from build123d import *

# Parameters (mm, degrees)
F0_W      = 150
F0_H      = 150
F1_DEPTH  = 25
F2_T      = -3
F3_R      = 6.25
F4_DEPTH  = 30
F5_R      = 6.25
F6_DEPTH  = 25
F7_R      = 6.25
F8_DEPTH  = 30
F9_R      = 6.25
F10_DEPTH = 30


with BuildPart() as f1:
    # F0 (on Front) → F1 (new body)
    with BuildSketch(Plane.XZ):
        with Locations((-12.459678, 3.580103)):
            Rectangle(F0_W, F0_H)
    extrude(amount=F1_DEPTH)

    # F2
    f2_openings = [f1.faces().sort_by_distance(p)[0] for p in [
        (-12.459678, 0, 3.580103),
    ]]
    offset(amount=F2_T, openings=f2_openings)

    # F3 (on face) → F4 (join)
    with BuildSketch(Plane.XY.offset(78.580103)):
        with Locations((-74.959678, -12.5)):
            Circle(F3_R)
        with Locations((50.040322, -12.5)):
            Circle(F3_R)
    extrude(amount=F4_DEPTH)

    # F5 (on face) → F6 (cut)
    with BuildSketch(Plane(origin=(0, 0, -71.419897), x_dir=(1, 0, 0), z_dir=(0, 0, -1))):
        with Locations((-74.959678, 12.5)):
            Circle(F5_R)
        with Locations((50.040322, 12.5)):
            Circle(F5_R)
    extrude(amount=-F6_DEPTH, mode=Mode.SUBTRACT)

    # F7 (on face) → F8 (join)
    with BuildSketch(Plane(origin=(-87.459678, 0, 0), x_dir=(0, -1, 0), z_dir=(-1, 0, 0))):
        with Locations((12.5, 66.080103)):
            Circle(F7_R)
        with Locations((12.5, -58.919897)):
            Circle(F7_R)
    extrude(amount=F8_DEPTH)

    # F9 (on face) → F10 (cut)
    with BuildSketch(Plane.YZ.offset(62.540322)):
        with Locations((-12.5, 66.080103)):
            Circle(F9_R)
        with Locations((-12.5, -58.919897)):
            Circle(F9_R)
    extrude(amount=-F10_DEPTH, mode=Mode.SUBTRACT)


solid = f1.part
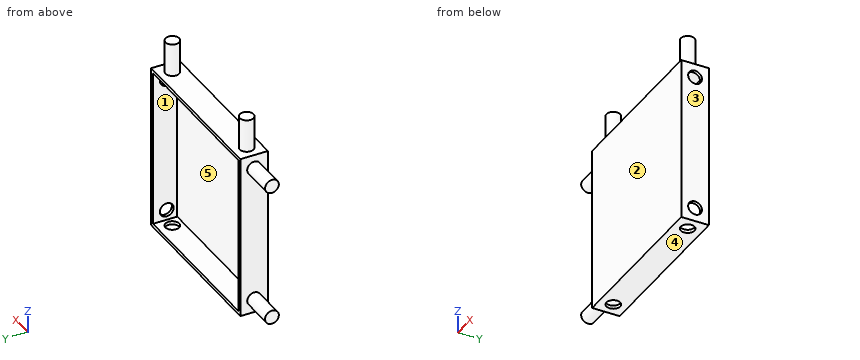
Source: CAD feature listing. Evaluate the final solid. Frame: model axes, mm. Face numbers are marked on the shaded views. A direction names the side the tool comes from. Give positions to 0.01 mm unless a question says otherwise; leave off trailing zeros. Write each loop counter-clockwise with the first axis right and the second up, starting at its lowest first coordinate (ties: lowest second). Pieces come first, ordered by that corner, then holes. Notation, with made-up numbers: M 35.5,-19 L 63.5,-19 A11 ccw 63.5,-7 Z; hole C -7.5,62.25 d3. An arc over 180 degrees is marked long. Return JSON: item names as keys, results as strings. Group by question number.
1) Set-up query: the marked faces 1 and 2. Return all of +Z, -Z, +X, -X, +Y, -Y with unobstructed straight access to the full face (end or side cutting, diameter ignored); none if empty.
2) Cut plane B-B, the plane x = -53.5. Output: boundary loops of the cut face in (y, z), plus the area to 3 significant figures.
3) Cut plane C-C, the plane y = -3.5. Output: boundary loops of the cut face in (x, z), plus the area to 3 significant figures.
4) Cut plane D-D, the plane y = -12.5. Give the number of separate pieces and of enclosed holes in the cut face, plus the area to 3 significant figures.
5) Pull-direction query (X, two-part tool) for the marked faces 3, 4 and 5; classes: pulls with the +X half, pulls with the -X half, needs draft (parallel to the pull), parting line crosses it, or undercut.
6) Cut plane A-A, the plane z = 88. Output: boundary loops of the cut face in (x, y), plus the area to 3 significant figures.
7) Material intervals for line 1 along Z through (x, y) = (61.8, -12.5); line 2 along X through (y, z) = (-12.5, -70.55); line 3 along Z through (x, y) = (-47, -12), sorted ascending. Write a range as [from, to].
8) Pin query (flat end, axial travel): P1, Ø12.5, axis at x = -22.5, y = -12.5, coming from the +Z side; P2, Ø7.5, axis at y = -12.5, z = -58.92, coming from the +X side; P3, Ø8, axis at x = 31.5, z = 53.5, coming from the +Y side. Return the tip coordinate at first contact, or that it passes through.
Recorded:
{
 "1": {"face 1": "+Y", "face 2": "+Z, -Z, +X, -X, -Y"},
 "2": {"outline": "M -25,-71.42 L 0,-71.42 L 0,-68.42 L -22,-68.42 L -22,75.58 L 0,75.58 L 0,78.58 L -25,78.58 Z", "area": "582 mm²"},
 "3": {"outline": "M -87.46,-71.42 L 62.54,-71.42 L 62.54,78.58 L -87.46,78.58 Z; hole M -84.46,-68.42 L 59.54,-68.42 L 59.54,75.58 L -84.46,75.58 Z", "area": "1,760 mm²"},
 "4": {"separate pieces": "4", "enclosed holes": "0", "area": "3,110 mm²"},
 "5": {"face 3": "pulls with the +X half", "face 4": "needs draft", "face 5": "undercut"},
 "6": {"outline": "C -74.96,-12.5 d12.5; C 50.04,-12.5 d12.5", "area": "245 mm²"},
 "7": {"line 1": "z = [-71.42, -65.17], [-52.67, 59.83], [72.33, 78.58]", "line 2": "x = [-87.46, -81.21], [-68.71, 43.79], [56.29, 62.54]", "line 3": "z = [-71.42, -68.42], [75.58, 78.58]"},
 "8": {"P1": "stops at z = 78.58", "P2": "stops at x = -84.46", "P3": "stops at y = -22"}
}
